The drawing under review shows one solid part. Ordinate dimensions are in mm from its lowest x, y, z. A direction names the side the tool comes from. Round coordinates to 2 decimals unless told otherwise and drop trailing zeros. Write each loop counter-clockwise with the first axis right and the second up, starting at its lowest first coordinate (ties: lowest second). Pieces come first, ordered by that corner, then holes.
Item 1: Add section D-D (z = 10.6). Give the boundary of the cut face in (x, y), plus the area to 3 significant figures.
Item 2: Add section A-A (y = 15). Give the boundary of the cut face in (x, z), plus the area to 3 significant figures.
Item 3: To check wall thickness, follow L1, parallel to X at y = 15, z = 0.4; L2, parallel to Z at x = 0.75, y = 5; L3, parallel to X at y = 34.5, z = 22. State the ranges of each line that lie inside material, in increasing order.
Item 4: Add section C-C (z = 20). Give the boundary of the cut face in (x, y), plus the area to 3 significant figures.
Item 5: Clearance check with flat-ended pins moving along their axes: pin 1 Ø11.5 at (y, z) = (20, 14) entering from +X; pin 2 Ø6.5 at (y, z) = (20, 20) entering from -X; pin 3 Ø5 at (x, y) = (33, 13) entering from +Z. State where each tip first meets the part, or that it passes through.
Item 6: Machinability: for the marked faces 1 and 2, which of the approach directions +Z, -Z, +X, -X, +Y, -Y give a long, thin tool a straight path to every point of the face, cutting with its end or side? Answer none if there is none.
Item 7: Add section B-B (x = 11.5). Give the boundary of the cut face in (y, z), plus the area to 3 significant figures.
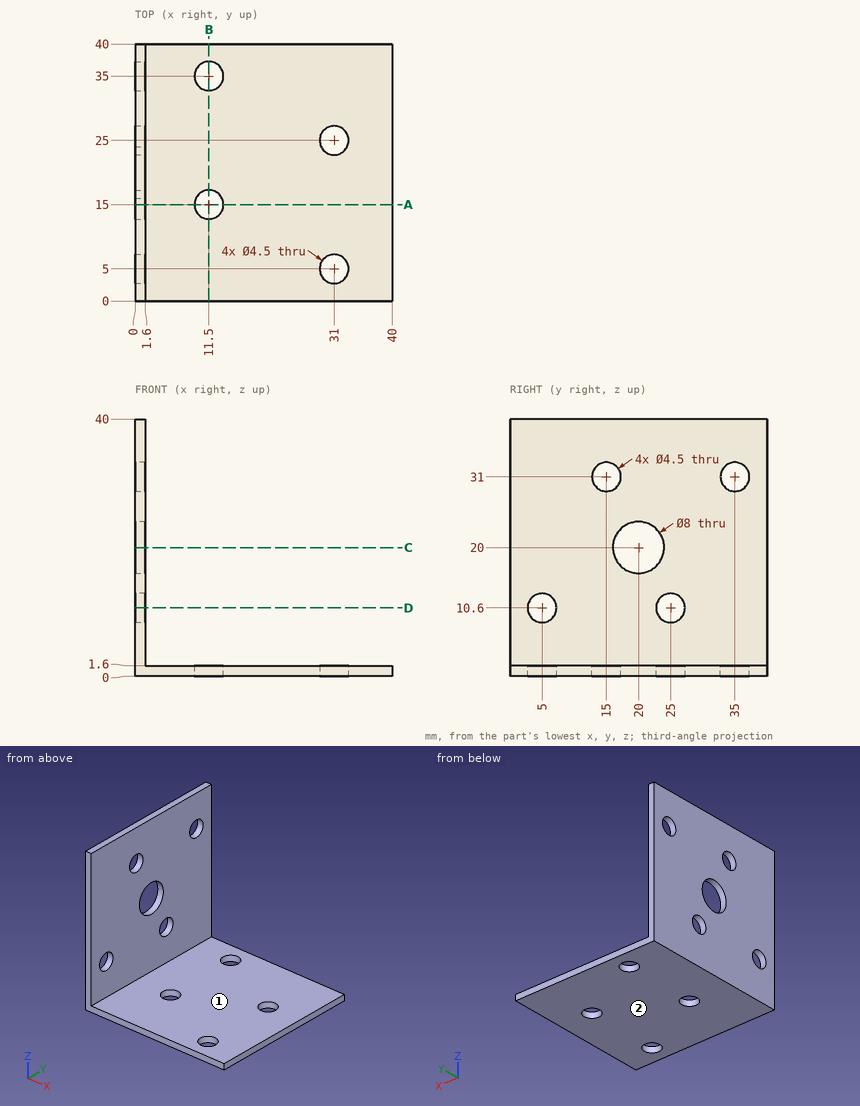
Numbers:
1. outline: (0, 0) - (1.6, 0) - (1.6, 2.75) - (0, 2.75) - close; (0, 7.25) - (1.6, 7.25) - (1.6, 22.75) - (0, 22.75) - close; (0, 27.25) - (1.6, 27.25) - (1.6, 40) - (0, 40) - close
1. area: 49.6 mm2
2. outline: (0, 0) - (9.25, 0) - (9.25, 1.6) - (1.6, 1.6) - (1.6, 28.75) - (0, 28.75) - close; (0, 33.25) - (1.6, 33.25) - (1.6, 40) - (0, 40) - close; (13.75, 0) - (40, 0) - (40, 1.6) - (13.75, 1.6) - close
2. area: 111 mm2
3. L1: x = 0 to 9.25, 13.75 to 40
3. L2: z = 0 to 8.35, 12.85 to 40
3. L3: x = 0 to 1.6
4. outline: (0, 0) - (1.6, 0) - (1.6, 16) - (0, 16) - close; (0, 24) - (1.6, 24) - (1.6, 40) - (0, 40) - close
4. area: 51.2 mm2
5. pin 1: stops at x = 1.6
5. pin 2: passes through
5. pin 3: stops at z = 1.6
6. face 1: +Z, +X, +Y, -Y
6. face 2: -Z, +X, -X, +Y, -Y
7. outline: (0, 0) - (12.75, 0) - (12.75, 1.6) - (0, 1.6) - close; (17.25, 0) - (32.75, 0) - (32.75, 1.6) - (17.25, 1.6) - close; (37.25, 0) - (40, 0) - (40, 1.6) - (37.25, 1.6) - close
7. area: 49.6 mm2
